The listing builds one solid part. Answer for the finished solid, in the listing's coordinates (mm). A direction names the side the tool comes from. Coordinates: 2 decimals unless noted, no trailing zeros. Order: outer loops, then holes, each group sorted by start corner. A loop starts at its lowest first (then second) coordinate and runs counter-clockwise, first axis right, second up. Notation, with made-up numbers: (-25, 33) - (-12, 33) arc R12 ccw to (-12, 44) - close; hole circle Ø4 at (-18.75, 19.5). An arc over 180 degrees is marked (long way). Use one line per item in the form item = value. Start each with the question number.
Item 1: Consider line 1 along Z through (x, y) = (13, -10); line 2 along Y through (x, z) = (9, 52); line 3 along Z through (x, y) = (34, 4.5). Determine where each line is inside the solid, lowest interval first. Write a range as [from, to].
Item 2: A tool of negligible diameter and unlimited length cuts with its end or side. For faces 5 (the flat face through (20, 0, 107)), 6 (the flat face through (20, 3, -74)), 7 (the cylindrical face through (37.972, 11.708, 88.229)), 8 (the flat face through (6, -10, 73)), from which of +Z, -Z, +X, -X, +Y, -Y can it reach the whole face along a straight path? Write none if from no direction.
Item 3: Section D-D, the plane z = 30.5 is taken. Write down the section's boundary in (x, y).
Item 4: Section A-A, the plane z = -47.5 is taken. Write down the section's boundary in (x, y), and give its area (3 significant figures).
Item 5: Each of these flat-tipped pins is pushed along its axis until it touches: pin 1 Ø2 at (y, z) = (0, 69) entering from -X; pin 2 Ø5 at (x, z) = (14, 65) entering from -Y; pin 3 Ø1.6 at (x, y) = (35.5, -10) entering from +Z. Where does it stop, or does it pass through?
Item 6: Section C-C, the plane x = 27 is taken. Write down the section's boundary in (y, z), and give its area (3 significant figures).
Item 7: Section B-B, the plane y = -6.5 is taken. Write down the section's boundary in (x, z), and give its area (3 significant figures).
Item 8: The mould has two halves that part along X. Classify faces 1 (the flat face through (20, 0, 41)), 2 (the flat face through (20, -20, 84)), 3 (the flat face through (20, 0, -93)), 4 (the flat face through (40, 14, 16)): released by +X, released by -X, zero draft, split by the parting line, or undercut.
from build123d import *

# Parameters (mm, degrees)
BOSS_EXTRUDE1_DEPTH = 40
CUT_EXTRUDE2_DEPTH  = 4
FILLET6_R           = 10
FILLET7_R           = 5
BOSS_EXTRUDE2_DEPTH = 20
BOSS_EXTRUDE3_DEPTH = 14


with BuildPart() as part:
    # Sketch1 → Boss-Extrude1 (new body)
    with BuildSketch(Plane(origin=(0, 0, 0), x_dir=(0, 0, -1), z_dir=(1, 0, 0))):
        Polygon((0, 0), (-130, 0), (-130, 5), (-100.000366453, 5.148280317), (-89.750475128, 15.5), (114, 15.5), (114, 0), (74, 0), (74, 6), (0, 6), align=None)
    extrude(amount=BOSS_EXTRUDE1_DEPTH)

    # Sketch6 → Cut-Extrude2 (cut)
    with BuildSketch(Plane(origin=(40, 0, 0), x_dir=(0, 0, -1), z_dir=(1, 0, 0))):
        Polygon((-100.876178749, 0), (114, 0), (114, 12.5), (-88.499139427, 12.5), align=None)
    cut_extrude2 = extrude(amount=-CUT_EXTRUDE2_DEPTH, mode=Mode.SUBTRACT)

    # Mirror3: Cut-Extrude2 across plane
    add(cut_extrude2.mirror(Plane(origin=(20, 0, 0), x_dir=(0, 0, 1), z_dir=(1, 0, 0))), mode=Mode.SUBTRACT)

    # Fillet6
    fillet6_edges = [part.edges().sort_by_distance(p)[0] for p in [
        (38, 0, 100.876178749),
        (38, 12.5, 88.499139427),
        (2, 0, 100.876178749),
        (2, 12.5, 88.499139427),
    ]]
    fillet(fillet6_edges, radius=FILLET6_R)

    # Fillet7
    fillet7_edges = [part.edges().sort_by_distance(p)[0] for p in [
        (20, 5.148280317, 100.000366453),
        (20, 15.5, 89.750475128),
    ]]
    fillet(fillet7_edges, radius=FILLET7_R)

    # Sketch7 → Boss-Extrude2 (add)
    with BuildSketch(Plane.XZ):
        Polygon((36, 85), (4, 85), (4, 64), (6, 64), (6, 83), (34, 83), (34, 64), (36, 64), align=None)
    extrude(amount=BOSS_EXTRUDE2_DEPTH)

    # Sketch9 → Boss-Extrude3 (add)
    with BuildSketch(Plane.XZ):
        Polygon((4, -114), (36, -114), (36, -93), (34, -93), (34, -112), (6, -112), (6, -93), (4, -93), align=None)
    extrude(amount=BOSS_EXTRUDE3_DEPTH)


solid = part.part
Response:
q1.line_1 = [-114, -112], [83, 85]
q1.line_2 = [0, 15.5]
q1.line_3 = [-114, -74], [0, 130]
q2.face_5 = +Z, +X, -X, -Y
q2.face_6 = +X, -X, -Y
q2.face_7 = -Z, +X, -Y
q2.face_8 = -Y
q3.outline = (0, 12.5) - (4, 12.5) - (4, 0) - (36, 0) - (36, 12.5) - (40, 12.5) - (40, 15.5) - (0, 15.5) - close
q4.outline = (0, 12.5) - (4, 12.5) - (4, 6) - (36, 6) - (36, 12.5) - (40, 12.5) - (40, 15.5) - (0, 15.5) - close
q4.area = 328 mm2
q5.pin_1 = 4
q5.pin_2 = 0
q5.pin_3 = 85
q6.outline = (-20, 83) - (0, 83) - (0, 0) - (6, 0) - (6, -74) - (0, -74) - (0, -112) - (-14, -112) - (-14, -114) - (15.5, -114) - (15.5, 87.66) arc R5 ccw to (14.02, 91.22) - (6.62, 98.54) arc R5 cw to (5.14, 102.07) - (5, 130) - (0, 130) - (0, 85) - (-20, 85) - close
q6.area = 3,040 mm2
q7.outline = (4, -114) - (36, -114) - (36, -93) - (34, -93) - (34, -112) - (6, -112) - (6, -93) - (4, -93) - close; (4, 64) - (6, 64) - (6, 83) - (34, 83) - (34, 64) - (36, 64) - (36, 85) - (4, 85) - close
q7.area = 280 mm2
q8.face_1 = undercut
q8.face_2 = zero draft
q8.face_3 = undercut
q8.face_4 = released by +X
